from build123d import *

# Parameters (mm, degrees)
F3_DEPTH = 144.93975
F4_R     = 3.175
F4_R_2   = 6.35
F4_R_3   = 9.525
F5_DEPTH = 63.501


with BuildPart() as f1:
    # F0 (on Front) → F1 (revolve)
    with BuildSketch(Plane.XZ):
        Polygon((-134.863547, 56.873039), (-141.76375, 63.5), (-144.93875, 63.5), (-144.93875, 0), (-137.309231, 0), (-134.987864, 46.427336), (-128.961906, 40.64), (-127.306591, 55.88), (0, 55.88), (0, 63.5), (-134.14375, 63.5), align=None)
    revolve(axis=Axis((0, 0, 31.75), (0, 0, -1)))

    # F2 (on Front) → F3 (cut, through all)
    with BuildSketch(Plane.XZ):
        Polygon((-137.16, 38.1), (-137.16, 2.984619), (-135.404231, 38.1), align=None)
        Polygon((-135.404231, 38.1), (-137.16, 2.984619), (-137.16, 0), (0, 0), (137.16, 0), (137.16, 38.1), (0, 38.1), align=None)
    extrude(amount=F3_DEPTH, mode=Mode.SUBTRACT)

    # F4 (on Top) → F5 (cut, through all)
    with BuildSketch(Plane.XY):
        with Locations((19.05, 0)):
            Circle(F4_R)
        with Locations((13.470384, 13.470384)):
            Circle(F4_R)
        with Locations((0, 19.05)):
            Circle(F4_R)
        with Locations((-13.470384, 13.470384)):
            Circle(F4_R)
        with Locations((-19.05, 0)):
            Circle(F4_R)
        with Locations((-13.470384, -13.470384)):
            Circle(F4_R)
        with Locations((0, -19.05)):
            Circle(F4_R)
        with Locations((13.470384, -13.470384)):
            Circle(F4_R)
        with Locations((38.1, 0)):
            Circle(F4_R)
        with Locations((32.05176, 20.598415)):
            Circle(F4_R)
        with Locations((15.827312, 34.656979)):
            Circle(F4_R)
        with Locations((76.2, 0)):
            Circle(F4_R_2)
        with Locations((-5.422195, 37.712197)):
            Circle(F4_R)
        with Locations((-24.950194, 28.794059)):
            Circle(F4_R)
        with Locations((-36.556682, 10.73401)):
            Circle(F4_R)
        with Locations((-36.556682, -10.73401)):
            Circle(F4_R)
        with Locations((-24.950194, -28.794059)):
            Circle(F4_R)
        with Locations((-5.422195, -37.712197)):
            Circle(F4_R)
        with Locations((15.827312, -34.656979)):
            Circle(F4_R)
        with Locations((32.05176, -20.598415)):
            Circle(F4_R)
        with Locations((64.103519, 41.19683)):
            Circle(F4_R_2)
        with Locations((31.654624, 69.313958)):
            Circle(F4_R_2)
        with Locations((-10.844391, 75.424394)):
            Circle(F4_R_2)
        with Locations((-49.900388, 57.588118)):
            Circle(F4_R_2)
        with Locations((-73.113365, 21.468021)):
            Circle(F4_R_2)
        with Locations((-73.113365, -21.468021)):
            Circle(F4_R_2)
        with Locations((-49.900388, -57.588118)):
            Circle(F4_R_2)
        with Locations((-10.844391, -75.424394)):
            Circle(F4_R_2)
        with Locations((31.654624, -69.313958)):
            Circle(F4_R_2)
        with Locations((64.103519, -41.19683)):
            Circle(F4_R_2)
        Circle(F4_R)
        with Locations((111.125, 0)):
            Circle(F4_R_3)
        with Locations((106.623657, 31.30753)):
            Circle(F4_R_3)
        with Locations((93.484299, 60.078711)):
            Circle(F4_R_3)
        with Locations((72.771399, 83.982671)):
            Circle(F4_R_3)
        with Locations((46.162993, 101.082855)):
            Circle(F4_R_3)
        with Locations((15.814736, 109.993908)):
            Circle(F4_R_3)
        with Locations((-15.814736, 109.993908)):
            Circle(F4_R_3)
        with Locations((-46.162993, 101.082855)):
            Circle(F4_R_3)
        with Locations((-72.771399, 83.982671)):
            Circle(F4_R_3)
        with Locations((-93.484299, 60.078711)):
            Circle(F4_R_3)
        with Locations((-106.623657, 31.30753)):
            Circle(F4_R_3)
        with Locations((-111.125, 0)):
            Circle(F4_R_3)
        with Locations((-106.623657, -31.30753)):
            Circle(F4_R_3)
        with Locations((-93.484299, -60.078711)):
            Circle(F4_R_3)
        with Locations((-72.771399, -83.982671)):
            Circle(F4_R_3)
        with Locations((-46.162993, -101.082855)):
            Circle(F4_R_3)
        with Locations((-15.814736, -109.993908)):
            Circle(F4_R_3)
        with Locations((15.814736, -109.993908)):
            Circle(F4_R_3)
        with Locations((46.162993, -101.082855)):
            Circle(F4_R_3)
        with Locations((72.771399, -83.982671)):
            Circle(F4_R_3)
        with Locations((93.484299, -60.078711)):
            Circle(F4_R_3)
        with Locations((106.623657, -31.30753)):
            Circle(F4_R_3)
    extrude(amount=F5_DEPTH, mode=Mode.SUBTRACT)


solid = f1.part
Read the model definition and answer for the solid it produces. Units are mm, in the model's axes. A direction names the side the tool comes from. Give positions to 0.01 mm unless a question says otherwise; leave off trailing zeros. Loops run counter-clockwise (first coordinate to the right, second up) from the corner with the lowest first, then second, coordinate; pieces in that order, holes last. Notation, with made-up numbers: (42, 53) -> (60, 53) arc R17 ccw to (60, 66) -> close; hole circle Ø8 at (-34.5, 85.25). An arc over 180 degrees is marked (long way). Use a Markdown table: item, result.
Q1. Section A-A, the plane x = 76.2 is taken. Count the separate pieces of the cut face and the enclosed holes in it, then the cut area to 3 significant figures.
Solved:
| item | result |
|---|---|
| separate pieces | 4 |
| enclosed holes | 0 |
| area | 2,470 mm^2 |
Q2. Section B-B, the plane z = 34.5 is taken. Determine the outline of the cut face in (x, y), then the cut area to 3 significant figures.
Solved:
| item | result |
|---|---|
| outline | (-137.16, -46.84) -> (-137.16, 0) -> (-135.58, 0) arc R135.58 cw to (135.58, 0) -> (137.16, 0) -> (137.16, -46.84) arc R144.94 ccw (long way) to start |
| area | 4,610 mm^2 |
Q3. Determine the mould class of faces 3 (the face through (33, 135, 0)), 4 (the face through (-38.9, -8.59, 59.64)) for opening direction X: pulls with the +X half, pulls with the -X half, needs draft (parallel to the pull), parting line crosses it, or undercut.
Solved:
| item | result |
|---|---|
| face 3 | needs draft |
| face 4 | undercut |
Q4. Find the intervals of material crossed by line 1 along X through (y, z) = (-19.05, 58.25) (3 decimals); line 2 along Z through (x, y) = (16.5, 30.5); line 3 along X through (y, z) = (-30.5, 7), in increasing order.
Solved:
| item | result |
|---|---|
| line 1 | x = -143.681 to -134.959, -133.36 to -78.985, -67.242 to -3.175, 3.175 to 29.28, 34.824 to 133.36, 134.959 to 143.681 |
| line 2 | z = 55.88 to 63.5 |
| line 3 | x = -141.69 to -137.16, 137.16 to 141.69 |
Q5. A tool of negligible diameter and unlimited length cuts with its end or side. For faces 1 (the face through (30.828, -63.018, 59.637)), 2 (the face through (2, -27, 55.88)), from which of +Z, -Z, +X, -X, +Y, -Y can it reach the whole face along a straight path? Write none if from no direction.
Solved:
| item | result |
|---|---|
| face 1 | +Z, -Z |
| face 2 | -Z |
Q6. Section D-D, the plane z = 9 is taken. Determine the outline of the cut face in (x, y), then the cut area to 3 significant figures.
Solved:
| item | result |
|---|---|
| outline | (-137.16, -46.84) -> (-137.16, 0) -> (-136.86, 0) arc R136.86 cw to (136.86, 0) -> (137.16, 0) -> (137.16, -46.84) arc R144.94 ccw (long way) to start |
| area | 4,060 mm^2 |
Q7. Each of these flat-tipped pins is pushed along its axis until it touches: pin 1 (6 mm diameter, centred on x = -26, z = 52.5, fed in from +Y); pin 2 (12 mm diameter, centred on x = -86, z = 29, fed in from +Y); pin 3 (6 mm diameter, centred on y = -112.5, z = 37.5, fed in from +X). Where does it stop, or does it pass through?
Solved:
| item | result |
|---|---|
| pin 1 | stops at y = 143.1 |
| pin 2 | stops at y = 120.86 |
| pin 3 | stops at x = 94.89 |
Q8. Section C-C, the plane z = 50 is taken. Determine the outline of the cut face in (x, y), then the cut area to 3 significant figures.
Solved:
| item | result |
|---|---|
| outline | circle Ø289.88 at (0, 0); hole circle Ø255.89 at (0, 0) |
| area | 14,600 mm^2 |
